Design review of the part built by this model. Coordinates are the model's own, in mm. A direction names the side the tool comes from. Coordinates: 2 decimals unless noted, no trailing zeros. Loops run counter-clockwise (first coordinate to the right, second up) from the corner with the lowest first, then second, coordinate; pieces in that order, holes last. Notation, with made-up numbers: (12.5, 65) -> (56.5, 65) arc R30 cw to (56.5, 89) -> close; hole circle Ø5 at (69.5, -14). An arc over 180 degrees is marked (long way). Use CSV: the item, a comma, the result in double quotes.
```python
from build123d import *

# Parameters (mm, degrees)
F1_DEPTH       = 15
F3_DEPTH       = 8
F5_D           = 3.2
F5_CBORE_D     = 5.6
F5_CBORE_DEPTH = 3
F6_R           = 4.5
F7_DEPTH       = 5
F8_R           = 4
F9_DEPTH       = 0.5
F10_R          = 2.5
F11_DEPTH      = 2
F12_SIZE       = 0.49999
F14_DEPTH      = 6
F15_R          = 4


# Not quite as in the source:
# - a fillet or chamfer is up to 0.001 mm smaller than in the source, because OpenCascade refuses the exact size


with BuildPart() as f1:
    # F0 (on Top) → F1 (new body)
    with BuildSketch(Plane.XY):
        with BuildLine():
            Line((2, -15.7), (2, -6.1846584384))
            ThreePointArc((2, -6.1846584384), (6.437849506, 0.8967127402), (0.2337698218, 6.4957949221))
            Line((0.2337698218, 6.4957949221), (-16.5553616693, 7.1))
            Line((-16.5553616693, 7.1), (-21.0553616693, 19.2963109177))
            Line((-21.0553616693, 19.2963109177), (-26.6844282466, 17.2193878407))
            Line((-26.6844282466, 17.2193878407), (-20.5672701971, 0.6401075063))
            Line((-20.5672701971, 0.6401075063), (-9.8485109145, -2.7956722641))
            ThreePointArc((-9.8485109145, -2.7956722641), (-7.7878175435, -4.283505147), (-7, -6.7))
            Line((-7, -6.7), (-7, -15.7))
            ThreePointArc((-7, -15.7), (-2.5, -20.2), (2, -15.7))
        make_face()
    extrude(amount=F1_DEPTH)

    # F2 (on face) → F3 (cut)
    with BuildSketch(Plane.XY.offset(15)):
        with BuildLine():
            Line((2, -15.7), (2, -9.8489847192))
            ThreePointArc((2, -9.8489847192), (2.8265485956, 9.6443311347), (-7, -7.2112758927))
            Line((-7, -7.2112758927), (-7, -15.7))
            ThreePointArc((-7, -15.7), (-2.5, -20.2), (2, -15.7))
        make_face()
    extrude(amount=-F3_DEPTH, mode=Mode.SUBTRACT)

    # F5 (through all)
    with Locations(Plane.XY.offset(7)):
        with Locations((-2.5, -15.7)):
            CounterBoreHole(F5_D / 2, F5_CBORE_D / 2, F5_CBORE_DEPTH)

    # F6 (on face) → F7 (cut)
    with BuildSketch(Plane(origin=(0, 0, 0), x_dir=(1, 0, 0), z_dir=(0, 0, -1))):
        Circle(F6_R)
    extrude(amount=-F7_DEPTH, mode=Mode.SUBTRACT)

    # F8 (on face) → F9 (join)
    with BuildSketch(Plane.XY.offset(7)):
        Circle(F8_R)
    extrude(amount=F9_DEPTH)

    # F10 (on face) → F11 (cut)
    with BuildSketch(Plane.XY.offset(7.5)):
        Circle(F10_R)
    extrude(amount=-F11_DEPTH, mode=Mode.SUBTRACT)

    # F12 (size 0.5 in the source; OpenCascade refuses exactly that, so slightly less here)
    f12_edges = [f1.edges().sort_by_distance(p)[0] for p in [
        (-4, 0, 7.5),
    ]]
    chamfer(f12_edges, length=F12_SIZE)

    # F13 (on face) → F14 (cut, through all)
    with BuildSketch(Plane(origin=(-17.8949713968, -6.6026007232, 0), x_dir=(0.3461538462, -0.9381777629, 0), z_dir=(-0.9381777629, -0.3461538462, 0))):
        with BuildLine():
            Line((-15.6917642328, 15), (-21.0917642328, 15))
            Line((-21.0917642328, 15), (-21.0917642328, 11.3076696831))
            ThreePointArc((-21.0917642328, 11.3076696831), (-18.3917642328, 7), (-15.6917642328, 11.3076696831))
            Line((-15.6917642328, 11.3076696831), (-15.6917642328, 15))
        make_face()
    extrude(amount=-F14_DEPTH, mode=Mode.SUBTRACT)

    # F15
    f15_edges = [f1.edges().sort_by_distance(p)[0] for p in [
        (2, -6.184658, 3.5),
    ]]
    fillet(f15_edges, radius=F15_R)


solid = f1.part
```
Item 1: To check wall thickness, follow line 1 along Y through (x, z) = (0, 6.7); line 2 along Y through (x, z) = (3, 0.75); line 3 along Y through (x, z) = (0, 1.75). State the ranges of each line that lie inside material, in increasing order.
Checked values:
line 1,"-19.44 to -16.96, -14.44 to -2.5, 2.5 to 6.5"
line 2,"-5.97 to -3.35, 3.35 to 5.77"
line 3,"-19.44 to -4.5, 4.5 to 6.5"
Item 2: Add section B-B (z = 10). Give the boundary of the cut face in (x, y).
Checked values:
outline,"(-26.68, 17.22) -> (-25.3, 13.47) -> (-19.67, 15.54) -> (-21.06, 19.3) -> close; (-23.22, 7.84) -> (-20.57, 0.64) -> (-9.85, -2.8) arc R4.1 cw to (-9.63, -2.87) arc R10.05 cw to (-7.43, 6.77) -> (-16.56, 7.1) -> (-17.59, 9.91) -> close"
Item 3: Clearance check with flat-ended pins moving along their axes: pin 1 (1 mm diameter, centred on y = 8.5, z = 3, fed in from -X); pin 2 (1 mm diameter, centred on y = 9, z = 13, fed in from +X); pin 3 (1.5 mm diameter, centred on x = -3.5, y = 2.5, fed in from +Z). State where each tip first meets the part, or that it passes through.
Checked values:
pin 1,"x = -23.65"
pin 2,"x = -17.07"
pin 3,"z = 7.45"
Item 4: Draft analysis for pull direction X (two halves, no side actions). For faces 1 (the face through (-2, -7, 7)), 2 (the face through (-23.83, 18.272, 7.395)), 3 (the face through (-22.42, 14.21, 13.18)), 4 (the face through (0, 0, 5)), state which applies: pulls with the +X half, pulls with the -X half, needs draft (parallel to the pull), parting line crosses it, or undercut.
Checked values:
face 1,"undercut"
face 2,"pulls with the -X half"
face 3,"pulls with the +X half"
face 4,"undercut"
Item 5: Add section A-A (z = 6). Give the boundary of the cut face in (x, y).
Checked values:
outline,"(-26.68, 17.22) -> (-20.57, 0.64) -> (-9.85, -2.8) arc R4.1 cw to (-7, -6.7) -> (-7, -15.7) arc R4.5 ccw to (2, -15.7) -> (2, -8.62) arc R4 cw to (3.71, -5.33) arc R6.5 ccw to (0.23, 6.5) -> (-16.56, 7.1) -> (-21.06, 19.3) -> close; hole circle Ø5.6 at (-2.5, -15.7); hole circle Ø5 at (0, 0)"
Item 6: Add section D-D (z = 12.5). Give the boundary of the cut face in (x, y), then the cut area to 3 significant figures.
Checked values:
outline,"(-26.68, 17.22) -> (-25.2, 13.19) -> (-19.57, 15.26) -> (-21.06, 19.3) -> close; (-23.33, 8.12) -> (-20.57, 0.64) -> (-9.85, -2.8) arc R4.1 cw to (-9.63, -2.87) arc R10.05 cw to (-7.43, 6.77) -> (-16.56, 7.1) -> (-17.7, 10.2) -> close"
area,"138 mm^2"
Item 7: Machinability: for faces 5 (the face through (-20.552, 9.143, 13.128)), 6 (the face through (-0.54, -2.44, 6.51)), 7 (the face through (-7, -11, 3)), which of the approach directions +Z, -Z, +X, -X, +Y, -Y give a long, thin tool a straight path to every point of the face, cutting with its end or side? Answer none if there is none.
Checked values:
face 5,"+Z, -X"
face 6,"+Z"
face 7,"+Z, -Z, -X, -Y"
Item 8: Add section C-C (z = 1.25). Give the boundary of the cut face in (x, y).
Checked values:
outline,"(-26.68, 17.22) -> (-20.57, 0.64) -> (-9.85, -2.8) arc R4.1 cw to (-7, -6.7) -> (-7, -15.7) arc R4.5 ccw to (2, -15.7) -> (2, -8.62) arc R4 cw to (3.71, -5.33) arc R6.5 ccw to (0.23, 6.5) -> (-16.56, 7.1) -> (-21.06, 19.3) -> close; hole circle Ø9 at (0, 0); hole circle Ø3.2 at (-2.5, -15.7)"
